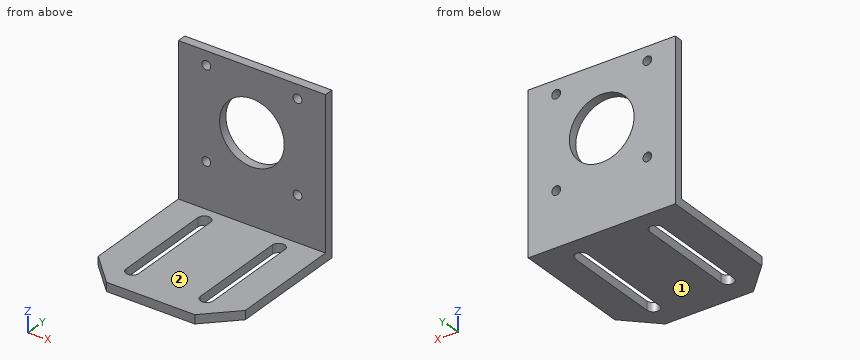
```python
from build123d import *

# Parameters (mm, degrees)
SKETCH1_W               = 50
SKETCH1_H               = 51
BOSS_EXTRUDE1_DEPTH     = 3
CUT_EXTRUDE_THIN1_DEPTH = 3
SKETCH4_W               = 50
SKETCH4_H               = 3
BOSS_EXTRUDE2_DEPTH     = 51
SKETCH5_R               = 11
CUT_EXTRUDE1_DEPTH      = 77.452599694
CUT_EXTRUDE2_DEPTH      = 77.452599694
CUT_EXTRUDE2_DEPTH_BACK = 77.452599694
SKETCH6_R               = 1.5


with BuildPart() as part:
    # Sketch1 → Boss-Extrude1 (new body)
    with BuildSketch(Plane.XY):
        Rectangle(SKETCH1_W, SKETCH1_H)
        with BuildLine():
            Line((-10.5, 17.5), (-10.5, -16.5))
            ThreePointArc((-10.5, -16.5), (-12.65, -18.65), (-14.8, -16.5))
            Line((-14.8, -16.5), (-14.8, 17.5))
            ThreePointArc((-14.8, 17.5), (-12.65, 19.65), (-10.5, 17.5))
        make_face(mode=Mode.SUBTRACT)
        with BuildLine():
            Line((10.5, 17.5), (10.5, -16.5))
            ThreePointArc((10.5, -16.5), (12.65, -18.65), (14.8, -16.5))
            Line((14.8, -16.5), (14.8, 17.5))
            ThreePointArc((14.8, 17.5), (12.65, 19.65), (10.5, 17.5))
        make_face(mode=Mode.SUBTRACT)
    extrude(amount=BOSS_EXTRUDE1_DEPTH)

    # Sketch3 → Cut-Extrude-Thin1 (cut)
    with BuildSketch(Plane(origin=(0, 0, 0), x_dir=(-1, 0, 0), z_dir=(0, 0, -1))):
        Polygon((-25, -15.5), (-15, -25.5), (-22.071067812, -32.571067812), (-32.071067812, -22.571067812), align=None)
        Polygon((15, -25.5), (25, -15.5), (32.071067812, -22.571067812), (22.071067812, -32.571067812), align=None)
    extrude(amount=-CUT_EXTRUDE_THIN1_DEPTH, mode=Mode.SUBTRACT)

    # Sketch4 → Boss-Extrude2 (add)
    with BuildSketch(Plane.XY.offset(3)):
        with Locations((0, 24)):
            Rectangle(SKETCH4_W, SKETCH4_H)
    extrude(amount=BOSS_EXTRUDE2_DEPTH)

    # Sketch5 → Cut-Extrude1 (cut, through all)
    with BuildSketch(Plane.XZ.offset(-22.5)):
        with Locations((0, 33)):
            Circle(SKETCH5_R)
    extrude(amount=-CUT_EXTRUDE1_DEPTH, mode=Mode.SUBTRACT)

    # Sketch6 → Cut-Extrude2 (cut, two sides: drawn at the far end of the back side and taken through both)
    with BuildSketch(Plane.XZ.offset(-22.5).offset(-CUT_EXTRUDE2_DEPTH_BACK)):
        with Locations((-15.5, 49.36722171)):
            Circle(SKETCH6_R)
        with Locations((-15.5, 18.36722171)):
            Circle(SKETCH6_R)
        with Locations((15.5, 18.36722171)):
            Circle(SKETCH6_R)
        with Locations((15.5, 49.36722171)):
            Circle(SKETCH6_R)
    extrude(amount=CUT_EXTRUDE2_DEPTH + CUT_EXTRUDE2_DEPTH_BACK, mode=Mode.SUBTRACT)


solid = part.part
```
Build history of the part. All positions in model axes, mm. Face numbers are marked on the shaded views. A direction names the side the tool comes from. Round coordinates to 2 decimals unless told otherwise and drop trailing zeros. Loops run counter-clockwise (first coordinate to the right, second up) from the corner with the lowest first, then second, coordinate; pieces in that order, holes last.
Item 1: Which spindle directions (+Z, -Z, +X, -X, +Y, -Y) get a long thin tool onto all of the face, cutting with end or side? Do the marked faces 1 and 2. Say none if no direction does.
Item 2: Drill centre lines: line 1 along Z through (x, y) = (15.5, 23.35); line 2 along Z through (x, y) = (0, 24); line 3 along Z through (x, y) = (-15, 23). Where is each one in solid material? Low to high.
Item 3: Pin check, flat tips, straight feed: P1, Ø12, axis at x = 15, y = -4.5, coming from the +Z side; P2, Ø3.5, axis at x = 15.5, z = 18.37, coming from the -Y side. Stop position of each tip, or through.
Item 4: Saw through at B-B (y = 10). List the corners of the cut face in (x, z).
Item 5: Saw through at C-C (z = 39). List the corners of the cut face in (x, y), then the cut area to 3 significant figures.
Item 6: Saw through at D-D (x = 0). List the corners of the cut face in (y, z), then the cut area to 3 significant figures.
Item 7: Saw through at A-A (x = -12.65). List the corners of the cut face in (y, z).
Worked answers:
1. face 1: -Z, +X, -X, +Y, -Y
1. face 2: +Z, +X, -X, -Y
2. line 1: z = 0 to 16.87, 19.87 to 47.87, 50.87 to 54
2. line 2: z = 0 to 22, 44 to 54
2. line 3: z = 0 to 16.95, 19.78 to 47.95, 50.78 to 54
3. P1: stops at z = 3
3. P2: stops at y = 22.5
4. outline: (-25, 0) - (-14.8, 0) - (-14.8, 3) - (-25, 3) - close; (-10.5, 0) - (10.5, 0) - (10.5, 3) - (-10.5, 3) - close; (14.8, 0) - (25, 0) - (25, 3) - (14.8, 3) - close
5. outline: (-25, 22.5) - (-9.22, 22.5) - (-9.22, 25.5) - (-25, 25.5) - close; (9.22, 22.5) - (25, 22.5) - (25, 25.5) - (9.22, 25.5) - close
5. area: 94.7 mm2
6. outline: (-25.5, 0) - (25.5, 0) - (25.5, 22) - (22.5, 22) - (22.5, 3) - (-25.5, 3) - close; (22.5, 44) - (25.5, 44) - (25.5, 54) - (22.5, 54) - close
6. area: 240 mm2
7. outline: (-25.5, 0) - (-18.65, 0) - (-18.65, 3) - (-25.5, 3) - close; (19.65, 0) - (25.5, 0) - (25.5, 54) - (22.5, 54) - (22.5, 3) - (19.65, 3) - close
